```python
from build123d import *

# Parameters (mm, degrees)
CUT_EXTRUDE_START   = -50
SKETCH_2_R          = 1.25
CUT_EXTRUDE_2_DEPTH = 6
SKETCH_4_W          = 12
SKETCH_4_H          = 12
EXTRUDE_1_DEPTH     = 5.4
FILLET_1_R          = 1
SKETCH_5_W          = 1.5
SKETCH_5_H          = 1
SKETCH_6_R          = 4.25
EXTRUDE_2_DEPTH     = 6
HOLE_WIZARD_M5_2_D  = 4.2


with BuildPart() as part:
    # 草图1 → 旋转1 (revolve)
    with BuildSketch(Plane.XY):
        Polygon((-8.5, 36), (-5.25, 36), (-5.25, 5), (-8.5, 5), (-8.5, 0), (-4.25, 0), (-4.25, 50), (-8.5, 50), align=None)
    revolve(axis=Axis((0, 0, 0), (0, 1, 0)))

    # 草图2 → 切除-拉伸2 (cut)
    with BuildSketch(Plane(origin=(0, 50, 0), x_dir=(1, 0, 0), z_dir=(0, 1, 0)).offset(CUT_EXTRUDE_START)):
        with Locations((0, 6.5)):
            Circle(SKETCH_2_R)
        with Locations((0, -6.5)):
            Circle(SKETCH_2_R)
        with Locations((-6.5, 0)):
            Circle(SKETCH_2_R)
        with Locations((6.5, 0)):
            Circle(SKETCH_2_R)
    extrude(amount=CUT_EXTRUDE_2_DEPTH, mode=Mode.SUBTRACT)

    # 草图4 → 凸台-拉伸1 (add)
    with BuildSketch(Plane(origin=(0, 50, 0), x_dir=(1, 0, 0), z_dir=(0, 1, 0))):
        Rectangle(SKETCH_4_W, SKETCH_4_H)
    extrude(amount=EXTRUDE_1_DEPTH)

    # 圆角1
    fillet_1_edges = [part.edges().sort_by_distance(p)[0] for p in [
        (6, 52.7, 6),
        (6, 52.7, -6),
        (-6, 52.7, -6),
        (-6, 52.7, 6),
    ]]
    fillet(fillet_1_edges, radius=FILLET_1_R)

    # 草图5 → 旋转2 (revolve)
    with BuildSketch(Plane.XY):
        with Locations((-9.25, 49.5)):
            Rectangle(SKETCH_5_W, SKETCH_5_H)
    revolve(axis=Axis((0, 0, 0), (0, 1, 0)))

    # 草图6 → 凸台-拉伸2 (add)
    with BuildSketch(Plane.XZ.offset(-50)):
        Circle(SKETCH_6_R)
    extrude(amount=EXTRUDE_2_DEPTH)

    # M5 螺纹孔2 (through all)
    with Locations(Plane(origin=(0, 55.4, 0), x_dir=(1, 0, 0), z_dir=(0, 1, 0))):
        with Locations((0, 0)):
            Hole(HOLE_WIZARD_M5_2_D / 2)


solid = part.part
```
Work out the finished part from the listing and answer in its coordinate system (mm). A direction names the side the tool comes from. Round coordinates to 2 decimals unless told otherwise and drop trailing zeros. Loops run counter-clockwise (first coordinate to the right, second up) from the corner with the lowest first, then second, coordinate; pieces in that order, holes last. Notation, with made-up numbers: M 60,-17.75 L 80,-17.75 A13 cw 80,-13.75 Z; hole C 18.5,81.25 d4. An arc over 180 degrees is marked long. Use CSV: the item, a comma, the result in double quotes.
Q1. Consider L1, parallel to Z at x = 0, y = 2.4; L2, parallel to Z at x = 0, y = 10; L3, parallel to X at y = 23, z = -0.25. Determine where each line is inside the solid, lowest interval first.
Determined:
L1,"-8.5 to -7.75, -5.25 to -4.25, 4.25 to 5.25, 7.75 to 8.5"
L2,"-5.25 to -4.25, 4.25 to 5.25"
L3,"-5.24 to -4.24, 4.24 to 5.24"
Q2. Section A-A, the plane z = -7.25 is taken. Determine the outline of the cut face in (x, y), then the cut area to 3 significant figures.
Determined:
outline,"M -6.89,49 L -4.44,49 L -4.44,36 L 4.44,36 L 4.44,49 L 6.89,49 L 6.89,50 L -6.89,50 Z; M -4.44,0 L -1,0 L -1,5 L -4.44,5 Z; M 1,0 L 4.44,0 L 4.44,5 L 1,5 Z"
area,"164 mm2"
Q3. Section B-B, the plane x = 6.5 is taken. Determine the outline of the cut face in (y, z), then the cut area to 3 significant figures.
Determined:
outline,"M 0,-5.48 L 5,-5.48 L 5,-1.25 L 0,-1.25 Z; M 0,1.25 L 5,1.25 L 5,5.48 L 0,5.48 Z; M 36,-5.48 L 49,-5.48 L 49,-7.6 L 50,-7.6 L 50,7.6 L 49,7.6 L 49,5.48 L 36,5.48 Z"
area,"200 mm2"
Q4. Section C-C, the plane y = 32 is taken. Determine the outline of the cut face in (x, z).
Determined:
outline,"C 0,0 d10.5; hole C 0,0 d8.5"
Q5. A tool of negligible diameter and unlimited length cuts with its end or side. For faces 1 (the flat face through (4, 5, 4)), 2 (the cylindrical face through (-0.27, 2.46, -5.28)), 3 (the flat face through (0, 53, 6)), from which of +Z, -Z, +X, -X, +Y, -Y can it reach the whole face along a straight path? Write none if from no direction.
Determined:
face 1,"none"
face 2,"-Y"
face 3,"+Z, +X, -X, +Y"
Q6. The mould has two halves that part along Z. Classify faces 4 (the cylindrical face through (5.699, 52.738, -5.715)), 5 (the cylindrical face through (-4.57, 2.465, 7.167)), 6 (the flat face through (-4, 36, 4)), 7 (the cylindrical face through (-7.75, 2.46, -0.05)): pulls with the +Z half, pulls with the -Z half, needs draft (parallel to the pull), parting line crosses it, or undercut.
Determined:
face 4,"pulls with the -Z half"
face 5,"parting line crosses it"
face 6,"needs draft"
face 7,"undercut"
Q7. Section D-D, the plane x = -3.75 is taken. Determine the outline of the cut face in (y, z).
Determined:
outline,"M 0,-7.63 L 5,-7.63 L 5,-3.67 L 36,-3.67 L 36,-7.63 L 49,-7.63 L 49,-9.27 L 50,-9.27 L 50,-6 L 55.4,-6 L 55.4,6 L 50,6 L 50,9.27 L 49,9.27 L 49,7.63 L 36,7.63 L 36,3.67 L 5,3.67 L 5,7.63 L 0,7.63 L 0,2 L 44,2 L 44,-2 L 0,-2 Z"
Q8. Each of these flat-tipped pins is pushed along its axis until it touches: pin 1 (6 mm diameter, centred on y = 13, z = 1, fed in from -X); pin 2 (10 mm diameter, centred on x = 3.5, z = 1.5, fed in from -Y); pin 3 (2 mm diameter, centred on y = 9, z = 4, fed in from +X); pin 4 (1.5 mm diameter, centred on x = 0, z = 6.5, fed in from -Y). Where does it stop, or does it pass through?
Determined:
pin 1,"x = -5.25"
pin 2,"y = 0"
pin 3,"x = 4.31"
pin 4,"y = 36"
